Autodesk Inventor part; units mm, degrees
ref_plane "Work Plane1" through (0, 0, 0) normal (0, 1, 0) x (1, 0, 0)
ref_plane "YZ Plane" through (0, 0, 0) normal (1, 0, 0) x (0, 1, 0)
ref_plane "XZ Plane" through (0, 0, 0) normal (0, 1, 0) x (-1, 0, 0)
sketch "Sketch1" plane through (0, 0, 0) normal (1, 0, 0) x (0, 1, 0)
  circle A0 centre (0, 0) radius 3
  circle A1 centre (0, 0) radius 1.6
  dimension "d0" = 3.2
  dimension "d1" = 6
extrude "Body" add sketch "Sketch1" along normal blind 0.4
sketch "Sketch2" plane through (0, 0, 0) normal (-1, 0, 0) x (0, 0, 1)
  circle A0 centre (0, 0) radius 1.6
  arc A1 (0.5118, 2.2423) -> (-0.5118, 2.2423) centre (0, 0) ccw
  line L0 (-0.356, 1.5599) -> (-0.5118, 2.2423)
  line L1 (-0.356, 1.5599) -> (0, 0) construction
  line L2 (0, 2.3) -> (0, 0) construction
  line L3 (0.356, 1.5599) -> (0.5118, 2.2423)
  line L4 (0.356, 1.5599) -> (0, 0) construction
  dimension "d6" = 4.6
  dimension "d7" = 12.857
extrude "Cut" cut sketch "Sketch2" along normal through all both and the other way through all contours A0 L0 A1 L3
fillet "Fillet1" radius 0.096 2 edges at (0.2, 2.2423, 0.5118) (0.2, 2.2423, -0.5118)
pattern_circular "Cuts" count 7 over 360 about axis through (-10, 0, 0) along (1, 0, 0) of "Cut", "Fillet1"
ref_plane "Work Plane1" through (0, 0, 0) normal (0, 1, 0) x (1, 0, 0)
equation "\"d0\" = SD1"
equation "\"d1\" = SD2"
equation "\"d2\" = SD"
equation "\"d6\" = 0.5 * SD2 + 0.5 * SD1"
equation "\"d8\" = SD"
equation "\"d10\" = 0.03 * SD1"
equation "\"SD1\" = 3.2"
equation "\"SD2\" = 6"
equation "\"SD\" = 0.4"
equation "\"NND\" = 3"
properties part number "DIN 6798 - J 3.2" material "Steel, Mild"
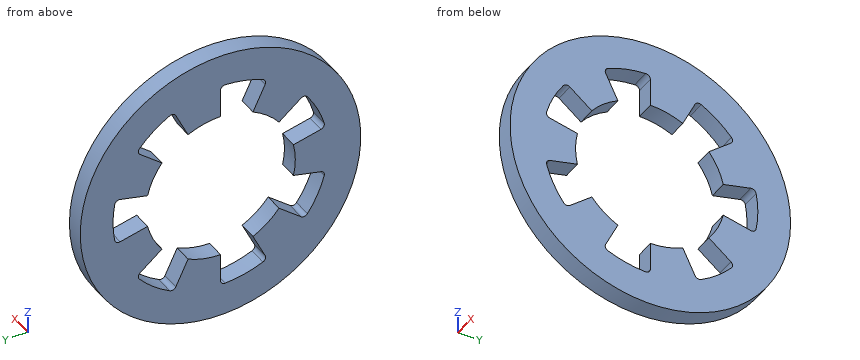
Work out the finished part from the listing and answer in its coordinate system (mm). Coordinates: 2 decimals unless noted, no trailing zeros. Write each loop counter-clockwise with the first axis right and the second up, starting at its lowest first coordinate (ties: lowest second). Pieces come first, ordered by that corner, then holes.
Q1. A cutting plane is placed at B-B, the plane z = -1.9. Give the vertices of the cut face in (x, y) (3 decimals).
Q2. A cutting plane is placed at D-D, the plane y = -2.05. Give the vertices of the cut face in (x, z).
Q3. This flat-tipped pin is pushed along its axis until it touches: pin 1 Ø1.5 at (y, z) = (-0.5, 1) entering from -X. Where does it stop, or does it pass through?
Q4. A cutting plane is placed at A-A, the plane z = 0. Give the vertices of the cut face in (x, y).
Q5. Find the intervals of material crossed by line 1 (Z direction, x = 0.15, y = 1.45); line 2 (Z direction, x = 0.1, y = -2); line 3 (Y direction, x = 0.35, z = -1.8), in increasing order.
Q6. A cutting plane is placed at C-C, the plane y = 0.25. Give the vertices of the cut face in (x, z), then the cut area to 3 significant figures.
Findings below:
1. outline: (0, -2.322) - (0.4, -2.322) - (0.4, -0.915) - (0, -0.915) - close; (0, 0) - (0.4, 0) - (0.4, 0.915) - (0, 0.915) - close; (0, 1.296) - (0.4, 1.296) - (0.4, 2.322) - (0, 2.322) - close
2. outline: (0, -2.19) - (0.4, -2.19) - (0.4, -1.04) - (0, -1.04) - close; (0, -0.47) - (0.4, -0.47) - (0.4, 0.47) - (0, 0.47) - close; (0, 1.04) - (0.4, 1.04) - (0.4, 2.19) - (0, 2.19) - close
3. pin 1: stops at x = 0
4. outline: (0, -3) - (0.4, -3) - (0.4, -1.6) - (0, -1.6) - close; (0, 2.3) - (0.4, 2.3) - (0.4, 3) - (0, 3) - close
5. line 1: z = -2.63 to -1.79, -1.16 to -0.68, 0.68 to 1.16, 1.79 to 2.63
5. line 2: z = -2.24 to -1.14, -0.46 to 0.46, 1.14 to 2.24
5. line 3: y = -2.4 to -0.87, 0 to 0.87, 1.43 to 2.4
6. outline: (0, -2.99) - (0.4, -2.99) - (0.4, -1.58) - (0, -1.58) - close; (0, 1.58) - (0.4, 1.58) - (0.4, 2.99) - (0, 2.99) - close
6. area: 1.13 mm2
